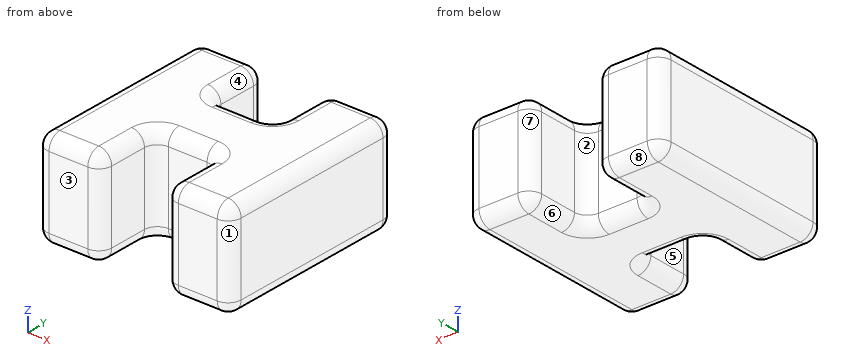
```python
from build123d import *

# Parameters (mm, degrees)
F0_W     = 10
F0_H     = 10
F1_DEPTH = 15
F2_R     = 2


with BuildPart() as f1:
    # F0 (on Top) → F1 (new body)
    with BuildSketch(Plane.XY):
        Polygon((0, 30), (0, 0), (10, 0), (10, 10), (10, 20), (10, 30), align=None)
        with Locations((15, 15)):
            Rectangle(F0_W, F0_H)
        Polygon((20, 20), (20, 10), (20, 0), (30, 0), (30, 30), (20, 30), align=None)
    extrude(amount=F1_DEPTH)

    # F2
    f2_edges = [f1.edges().sort_by_distance(p)[0] for p in [
        (0, 30, 7.5),
        (20, 30, 7.5),
        (0, 0, 7.5),
        (10, 0, 7.5),
        (5, 0, 0),
        (5, 0, 15),
        (20, 0, 7.5),
        (30, 0, 7.5),
        (25, 0, 0),
        (25, 0, 15),
        (10, 20, 7.5),
        (10, 30, 7.5),
        (10, 25, 0),
        (10, 25, 15),
        (20, 20, 7.5),
        (20, 25, 0),
        (20, 25, 15),
        (30, 30, 7.5),
        (25, 30, 0),
        (25, 30, 15),
        (30, 15, 15),
        (10, 10, 7.5),
        (10, 5, 0),
        (10, 5, 15),
        (5, 30, 0),
        (5, 30, 15),
        (15, 20, 15),
        (20, 10, 7.5),
        (15, 10, 0),
        (15, 10, 15),
        (20, 5, 15),
        (0, 15, 0),
        (0, 15, 15),
        (30, 15, 0),
        (20, 5, 0),
        (15, 20, 0),
    ]]
    fillet(f2_edges, radius=F2_R)


solid = f1.part
```
Here's how the part is built. I have some questions about the finished solid (model axes, mm). Face numbers are marked on the shaded views. A direction names the side the tool comes from. Coordinates: 2 decimals unless noted, no trailing zeros. Order: outer loops, then holes, each group sorted by start corner. A loop starts at its lowest first (then second) coordinate and runs counter-clockwise, first axis right, second up.
Item 1: If we section it at A-A, the plane y = 2.75: List the corners of the cut face in (x, z) for me, then the cut area to 3 significant figures.
Response values:
outline: (0, 2) arc R2 ccw to (2, 0) - (8, 0) arc R2 ccw to (10, 2) - (10, 13) arc R2 ccw to (8, 15) - (2, 15) arc R2 ccw to (0, 13) - close; (20, 2) arc R2 ccw to (22, 0) - (28, 0) arc R2 ccw to (30, 2) - (30, 13) arc R2 ccw to (28, 15) - (22, 15) arc R2 ccw to (20, 13) - close
area: 293 mm2
Item 2: I'm going to push flat-ended pins straight in: pin 1 Ø1.8 at (x, z) = (15, 9) entering from +Y; pin 2 Ø8 at (x, y) = (21, 20.5) entering from +Z; pin 3 Ø1.8 at (x, z) = (14.5, 10) entering from -Y. Where does each tip first touch, or does it pass through?
Response values:
pin 1: stops at y = 20
pin 2: stops at z = 15
pin 3: stops at y = 10
Item 3: If we section it at B-B, the plane z = 12.25: List the corners of the cut face in (x, y) for me, then the cut area to 3 significant figures.
Response values:
outline: (0, 2) arc R2 ccw to (2, 0) - (8, 0) arc R2 ccw to (10, 2) - (10, 8) arc R2 cw to (12, 10) - (18, 10) arc R2 cw to (20, 8) - (20, 2) arc R2 ccw to (22, 0) - (28, 0) arc R2 ccw to (30, 2) - (30, 28) arc R2 ccw to (28, 30) - (22, 30) arc R2 ccw to (20, 28) - (20, 22) arc R2 cw to (18, 20) - (12, 20) arc R2 cw to (10, 22) - (10, 28) arc R2 ccw to (8, 30) - (2, 30) arc R2 ccw to (0, 28) - close
area: 697 mm2
Item 4: Thinking about a two-plate mould opening in X: for the marked faces 1, 2 and 3, which applies, pulls with the +X half, pulls with the -X half, needs draft (parallel to the pull), parting line crosses it, or undercut?
Response values:
face 1: pulls with the +X half
face 2: undercut
face 3: needs draft
Item 5: I need wall thicknesses on probe 1 along X at (y, z) = (6.5, 10.5); probe 2 along X at (y, z) = (5.75, 14); probe 3 along Z at (x, y) = (21.75, 21.25). Which ranges of each line are inside material? Lowest first, please.
Response values:
probe 1: x = 0 to 10, 20 to 30
probe 2: x = 0.27 to 9.73, 20.27 to 29.73
probe 3: z = 0.01 to 14.99
Item 6: Which directions (+Z, -Z, +X, -X, +Y, -Y) give clear straight access to the entire face, cutting with the end or side of a thin tool? Please do the marked faces 4, 5, 6, 7 and 8.
Response values:
face 4: +Z, +Y
face 5: +Z, -Z, -Y
face 6: -Z, +Y
face 7: +Z, -Z, +Y
face 8: -Z, +X, -X, +Y
